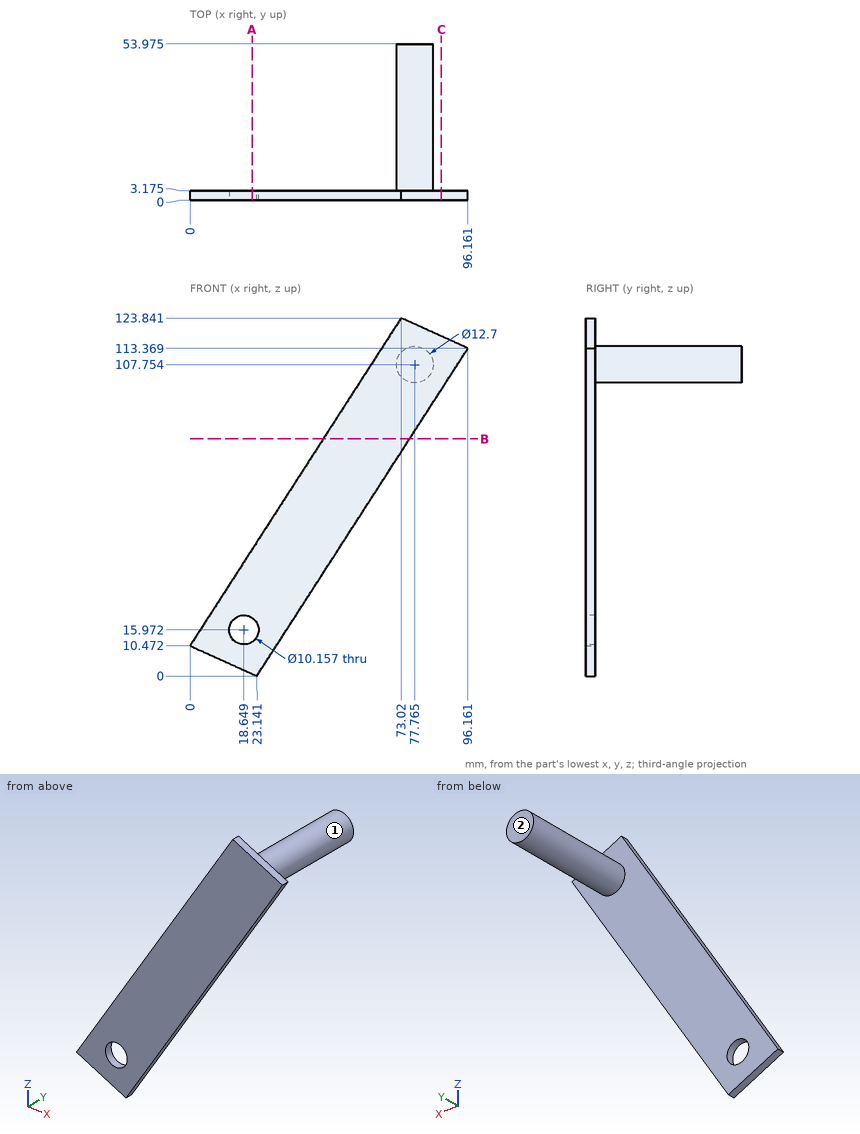
Design review of the part shown in the three views and the two pictorial views. Dimensions are in mm from the part's minimum x, y and z. A direction names the side the tool comes from. Round coordinates to 2 decimals unless told otherwise and drop trailing zeros. Loops run counter-clockwise (first coordinate to the right, second up) from the corner with the lowest first, then second, coordinate; pieces in that order, holes last.
(1) We need section C-C (x = 87). Give the boundary of the cut face in (y, z) (1 decimal).
Returned:
outline: (0, 99.1) - (3.2, 99.1) - (3.2, 117.5) - (0, 117.5) - close
(2) We need section A-A (x = 21.5). Give the boundary of the cut face in (y, z) (1 decimal).
Returned:
outline: (0, 0.7) - (3.2, 0.7) - (3.2, 11.8) - (0, 11.8) - close; (0, 20.2) - (3.2, 20.2) - (3.2, 43.9) - (0, 43.9) - close
(3) Wall thickness on line 1 along X through (y, z) = (6, 108); line 2 along X through (y, z) = (34, 106.5); line 3 along Z through (x, y) = (82, 50) (1 decimal): over which ranges is each line inside the solid? List them lowest first.
Returned:
line 1: x = 71.42 to 84.11
line 2: x = 71.54 to 83.99
line 3: z = 103 to 112.5
(4) Clearance check with flat-ended pins moving along their axes: P1, Ø5, axis at y = 43, z = 106.5, coming from the +X side (1 decimal); P2, Ø11.5, axis at x = 18.65, z = 15.97, coming from the +Y side (3 decimals). State where each tip first meets the part, or that it passes through.
Returned:
P1: stops at x = 84.1
P2: stops at y = 3.175
(5) We need section B-B (z = 82). Give the boundary of the cut face in (x, y) (1 decimal).
Returned:
outline: (46.1, 0) - (76, 0) - (76, 3.2) - (46.1, 3.2) - close
(6) Tool access review of the marked faces 1 and 2: name each direction out of +Z, -Z, +X, -X, +Y, -Y from which nothing blocks a thin tool from reaching the whole face with its end or side.
Returned:
face 1: +Y
face 2: +Z, -Z, +X, -X, +Y
